Study the drawing (mm; zero at the part's minimum x, y, z) and answer. Give positions to 0.01 mm unless a question says otherwise; leave off trailing zeros. Order: outer loops, then holes, each group sorted by start corner. A loop starts at its lowest first (then second) coordinate and runs counter-clockwise, first axis right, second up. Notation, with made-up numbers: (-20, -32.75) - (3, -32.75) arc R35 ccw to (3, 0.25) - close; hole circle Ø4 at (55.5, -23). An arc over 180 degrees is marked (long way). Return JSON: item names as keys, results as strings.
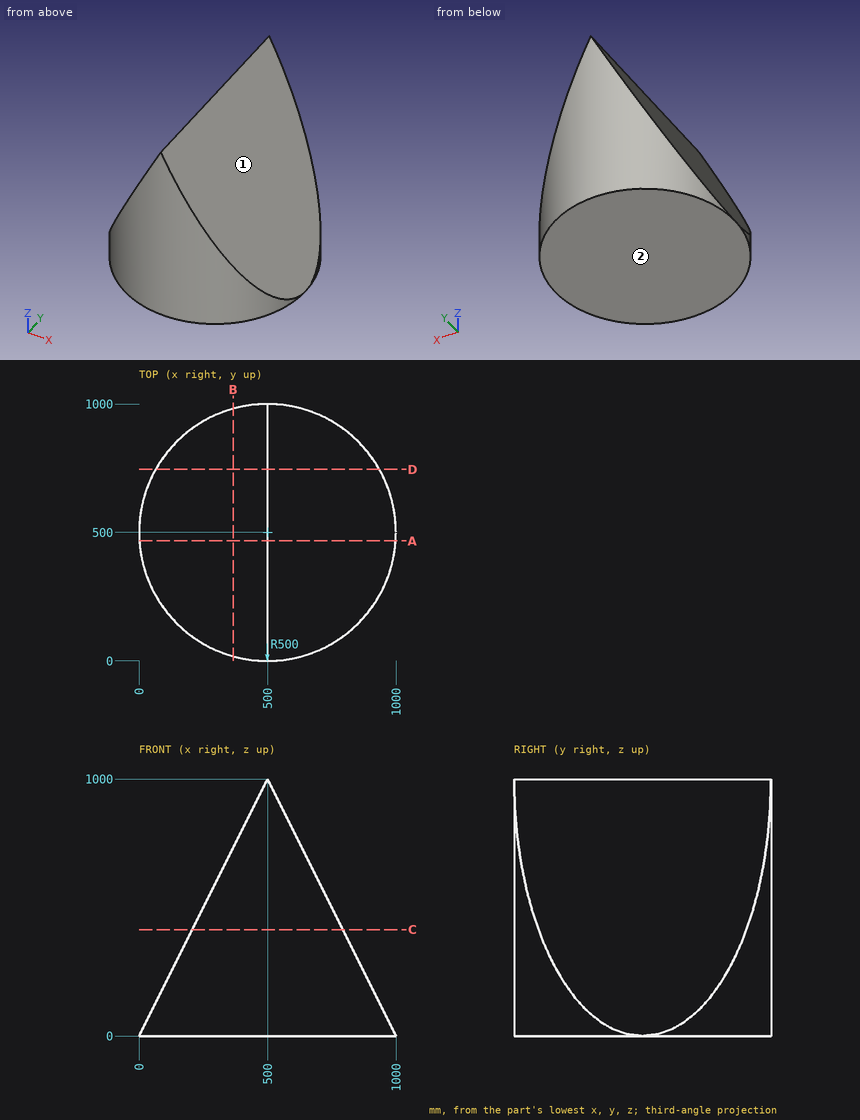
Q1. A cutting plane is placed at A-A (y = 467.5). Write down the section's boundary in (x, z), and give its area (3 significant figures).
Values:
{"outline": "(1.06, 0) - (998.94, 0) - (998.94, 2.11) - (500, 1000) - (1.06, 2.11) - close", "area": "500,000 mm²"}
Q2. A cutting plane is placed at C-C (z = 413.5). Write down the section's boundary in (x, y), and give its area (3 significant figures).
Values:
{"outline": "(206.75, 95.03) arc R500 ccw to (793.25, 95.03) - (793.25, 904.97) arc R500 ccw to (206.75, 904.97) - close", "area": "551,000 mm²"}
Q3. Consider L1, parallel to Y at x = 515.5, z = 513.5; L2, parallel to Y at x = 203, z = 358; L3, parallel to X at y = 286, z = 616. Determine where each line is inside the solid, lowest interval first.
Values:
{"L1": "y = 0.24 to 999.76", "L2": "y = 97.77 to 902.23", "L3": "x = 308 to 692"}
Q4. A cutting plane is placed at B-B (x = 366.5). Write down the section's boundary in (y, z), and give its area (3 significant figures).
Values:
{"outline": "(18.15, 0) - (981.85, 0) - (981.85, 733) - (18.15, 733) - close", "area": "706,000 mm²"}
Q5. Given pin 1 (1.5 mm diameter, centred on y = 798, z = 597, fed in from +X) (3 decimals); pin 2 (4 mm diameter, centred on y = 593, z = 411.5, fed in from -X); pin 3 (1 mm diameter, centred on x = 822.5, y = 677.5, fed in from +Z), each flat-ended and moving along its own axis, determine where each tip first touches the part or whether it passes through.
Values:
{"pin 1": "stops at x = 701.875", "pin 2": "stops at x = 204.75", "pin 3": "stops at z = 356"}
Q6. Determine the mould class of the marked faces 1 and 2 for opening direction Z: released by +Z, released by -Z, zero draft, split by the parting line, or undercut.
Values:
{"face 1": "released by +Z", "face 2": "released by -Z"}
Q7. A cutting plane is placed at D-D (y = 746). Write down the section's boundary in (x, z), and give its area (3 significant figures).
Values:
{"outline": "(64.7, 0) - (935.3, 0) - (935.3, 129.4) - (500, 1000) - (64.7, 129.4) - close", "area": "492,000 mm²"}
